```python
from build123d import *

# Parameters (mm, degrees)
SKETCH_R              = 1.6
PAD_DEPTH             = 3
POLARPATTERN_COUNT    = 3
POCKET_DEPTH          = 316.40103
POLARPATTERN001_COUNT = 3
CHAMFER_SIZE          = 1
FILLET_R              = 3
SKETCH066_R           = 1.6
POCKET032_DEPTH       = 3.001


with BuildPart() as part:
    # Sketch → Pad (new body)
    with BuildSketch(Plane.XY):
        Polygon((0, 0), (-47.320508, 27.320508), (-54.641016, 14.641016), (-49.641016, 5.980762), (-58.30127, 0.980762), (-28.30127, -50.980762), (-19.641016, -45.980762), (-14.641016, -54.641016), (0, -54.641016), align=None)
        with Locations((-48.971143, -5.179492)):
            Circle(SKETCH_R, mode=Mode.SUBTRACT)
        with Locations((-28.971143, -39.820508)):
            Circle(SKETCH_R, mode=Mode.SUBTRACT)
    pad = extrude(amount=PAD_DEPTH)

    # PolarPattern: Pad ×3 about axis
    polarpattern_axis = Axis((0, 0, 0), (0, 0, 1))
    for i in range(1, POLARPATTERN_COUNT):
        add(pad.rotate(polarpattern_axis, i * 360 / POLARPATTERN_COUNT))

    # Sketch001 → Pocket (cut, through all)
    with BuildSketch(Plane.XY):
        Polygon((-25.669873, 14.820508), (-34.669873, -0.767949), (-18, -29.641016), (0, -29.641016), (0, 0), align=None)
    pocket = extrude(amount=POCKET_DEPTH, mode=Mode.SUBTRACT)

    # PolarPattern001: Pocket ×3 about axis
    polarpattern001_axis = Axis((0, 0, 0), (0, 0, 1))
    for i in range(1, POLARPATTERN001_COUNT):
        add(pocket.rotate(polarpattern001_axis, i * 360 / POLARPATTERN001_COUNT), mode=Mode.SUBTRACT)

    # Chamfer
    chamfer_edges = [part.edges().sort_by_distance(p)[0] for p in [
        (-54.641016, 14.641016, 1.5),
        (-40, 40, 1.5),
        (-30, 50, 1.5),
        (30, 50, 1.5),
        (40, 40, 1.5),
        (54.641016, 14.641016, 1.5),
        (58.30127, 0.980762, 1.5),
        (28.30127, -50.980762, 1.5),
        (14.641016, -54.641016, 1.5),
        (-14.641016, -54.641016, 1.5),
        (-28.30127, -50.980762, 1.5),
        (-58.30127, 0.980762, 1.5),
    ]]
    chamfer(chamfer_edges, length=CHAMFER_SIZE)

    # Fillet
    fillet_edges = [part.edges().sort_by_distance(p)[0] for p in [
        (-16.669873, 30.408965, 1.5),
        (18, -29.641016, 1.5),
        (-18, -29.641016, 1.5),
        (34.669873, -0.767949, 1.5),
        (16.669873, 30.408965, 1.5),
        (-34.669873, -0.767949, 1.5),
    ]]
    fillet(fillet_edges, radius=FILLET_R)

    # Sketch066 (on Binder) → Pocket032 (cut, through all)
    with BuildSketch(Plane(origin=(0, 0, 3), x_dir=(1, 0, 0), z_dir=(0, 0, -1))):
        with Locations((-24.348373, 30.5)):
            Circle(SKETCH066_R)
        with Locations((38.587961, 5.836309)):
            Circle(SKETCH066_R)
        with Locations((-14.239588, -36.336309)):
            Circle(SKETCH066_R)
    extrude(amount=POCKET032_DEPTH, mode=Mode.SUBTRACT)


solid = part.part
```
Build history of the part. All positions in model axes, mm. A direction names the side the tool comes from. Round coordinates to 2 decimals unless told otherwise and drop trailing zeros. Loops run counter-clockwise (first coordinate to the right, second up) from the corner with the lowest first, then second, coordinate; pieces in that order, holes last.
Item 1: Which spindle directions (+Z, -Z, +X, -X, +Y, -Y) get a long thin tool onto all of the face, cutting with end or side? Do faces 1 (the face through (35, 40, 1)), 2 (the face through (-23.59, -48.26, 1.48)), 3 (the face through (-26.44, -15.02, 1.48)). Say none if no direction does.
Item 2: Saw through at A-A (y = 45). List the corners of the cut face in (x, z).
Item 3: Two-plate mould, pull along Y, no slides. Class faces 4 (the face through (29.83, -38.47, 1.48)), 5 (the face through (6, -32, 3)), 6 (the face through (0, 50, 1)), 7 (the face through (-16.419, 30.018, 1.521)): released by +Y, released by -Y, zero draft, split by the parting line, or undercut.
Item 4: Drill centre lines: line 1 along Y through (x, z) = (-6.5, 2.65); line 2 along Y through (x, z) = (20, 1.4); line 3 along X through (y, z) = (-4, 1.35). Where is each one in solid material? Low to high.
Item 5: Saw through at C-C (y = 10.5). List the corners of the cut face in (x, z), then the cut area to 3 significant figures.
Item 6: Saw through at B-B (x = -3). List the corners of the cut face in (y, z), then the cut area to 3 significant figures.
Item 7: Saw through at D-D (z = 1.75). State how many separate pieces and enclosed holes the cut face has, then the cut area to 3 significant figures.
Worked answers:
1. face 1: +Z, -Z, +X, +Y
1. face 2: +Z, -Z, -Y
1. face 3: +Z, -Z
2. outline: (-30, 0) - (-21.6, 0) - (-21.6, 3) - (-30, 3) - close; (-18.4, 0) - (18.4, 0) - (18.4, 3) - (-18.4, 3) - close; (21.6, 0) - (30, 0) - (30, 3) - (21.6, 3) - close
3. face 4: undercut
3. face 5: zero draft
3. face 6: released by +Y
3. face 7: undercut
4. line 1: y = -54.64 to -29.64, 30.41 to 50
4. line 2: y = -46.19 to -26.18, 24.64 to 43.4, 46.6 to 50
4. line 3: x = -55.43 to -50.05, -47.89 to -32.8, 32.8 to 47.89, 50.05 to 55.43
5. outline: (-52.25, 0) - (-28.16, 0) - (-28.16, 3) - (-52.25, 3) - close; (28.16, 0) - (52.25, 0) - (52.25, 3) - (28.16, 3) - close
5. area: 145 mm2
6. outline: (-54.64, 0) - (-29.64, 0) - (-29.64, 3) - (-54.64, 3) - close; (30.41, 0) - (50, 0) - (50, 3) - (30.41, 3) - close
6. area: 134 mm2
7. separate pieces: 1
7. enclosed holes: 10
7. area: 5,800 mm2
